For this review, take the finished solid that the model builds, in its own axes (mm). A direction names the side the tool comes from. Round coordinates to 2 decimals unless told otherwise and drop trailing zeros. Write each loop counter-clockwise with the first axis right and the second up, starting at its lowest first coordinate (ties: lowest second). Pieces come first, ordered by that corner, then holes. Notation, with made-up numbers: M -5.5,4 L 19.5,4 A30 ccw 19.5,40 Z; hole C 68,76.5 d7. An arc over 180 degrees is marked long. Use one line per item in the form item = value. Start each with the question number.
Item 1: Add section D-D (z = -2.2). State the section outline as (x, y) points, and give its area (3 significant figures).
Item 2: For faces 1 (the flat face through (1.25, 16, 0)), 2 (the flat face through (0, 0, 0)), 3 (the flat face through (1.2, 14, 1.2)), list the 3-axis set-ups (+Z, -Z, +X, -X, +Y, -Y) from which the entire face can be reached by the end or side of a thin tool; tool diameter is ignored.
Item 3: Add section A-A (z = 0). State the section outline as (x, y) points, and give its area (4 significant figures).
Item 4: For line 1 (Y direction, x = 0.55, z = 0.5); line 2 (Y direction, x = -0.8, z = -1.85); line 3 (X direction, y = 13, z = 0.4), list the stretches that pass through material, from the lowest coordinate up. Write a range as [from, to].
Item 5: Add section B-B (y = 4.75). State the section outline as (x, z) points, and give its area (3 significant figures).
Item 6: Add section C-C (x = -1.9). State the section outline as (y, z) points, and give its area (3 significant figures).
Item 7: Draft analysis for pull direction X (two halves, no side actions). For faces 4 (the flat face through (0.616, 16.014, -1.088)), 5 (the flat face through (-1.25, 16, 0)), 6 (the flat face through (0.6, 17, -1.3)), 7 (the cylindrical face through (1.5, 7.16, -0.07)), state which applies: released by +X, released by -X, zero draft, split by the parting line, or undercut.
Item 8: For P1, Ø1.5, axis at y = 8, z = 2, coming from the +X side; P2, Ø1, axis at y = 4, z = -0.5, coming from the -X side, all flat-tipped, find the tip position at first contact; note any pin that passes through.
Autodesk Inventor part; units mm, degrees
ref_plane "YZ Plane" through (0, 0, 0) normal (1, 0, 0) x (0, 1, 0)
ref_plane "XZ Plane" through (0, 0, 0) normal (0, 1, 0) x (-1, 0, 0)
ref_plane "XY Plane" through (0, 0, 0) normal (0, 0, 1) x (1, 0, 0)
sketch "Sketch1" plane through (0, 0, 0) normal (0, 1, 0) x (-1, 0, 0)
  circle A0 centre (0, 0) radius 1.5
  dimension "d0" = 3
extrude "Extrusion1" add sketch "Sketch1" along normal blind 14
sketch "Sketch2" plane through (0, 14, 0) normal (0, 1, 0) x (1, 0, 0)
  circle A0 centre (0, 0) radius 1.5
  circle A1 centre (0, 0) radius 2.75
  dimension "d3" = 5.5
extrude "Extrusion2" add sketch "Sketch2" along normal blind 3 contours A0 | A1
sketch "Sketch3" plane through (0, 17, 0) normal (0, 1, 0) x (1, 0, 0)
  circle A0 centre (0, 0) radius 2.75
  line L0 (0, 1.4434) -> (1.25, 0.7217)
  line L1 (1.25, 0.7217) -> (1.25, -0.7217)
  line L2 (1.25, -0.7217) -> (0, -1.4434)
  line L3 (0, -1.4434) -> (-1.25, -0.7217)
  line L4 (-1.25, -0.7217) -> (-1.25, 0.7217)
  line L5 (-1.25, 0.7217) -> (0, 1.4434)
  dimension "d6" = 2.5
extrude "Extrusion3" cut sketch "Sketch3" against normal blind 2 contours L0 L1 L2 L3 L4 L5
thread "Thread1"
chamfer "Chamfer1" distance 0.5 angle 45 1 edges at (1.5, 0, 0)
properties part number "M3x14SHCS"
Calculated:
q1.outline = M -1.65,14 L 1.65,14 L 1.65,17 L -1.65,17 Z
q1.area = 9.90 mm^2
q2.face_1 = +Y
q2.face_2 = +Z, -Z, +X, -X, -Y
q2.face_3 = -Y
q3.outline = M -2.75,14 L -1.5,14 L -1.5,0.5 L -1,0 L 1,0 L 1.5,0.5 L 1.5,14 L 2.75,14 L 2.75,17 L 1.25,17 L 1.25,15 L -1.25,15 L -1.25,17 L -2.75,17 Z
q3.area = 53.25 mm^2
q4.line_1 = [0, 15]
q4.line_2 = [14, 17]
q4.line_3 = [-1.45, 1.45]
q5.outline = C 0,0 d3
q5.area = 7.07 mm^2
q6.outline = M 14,-1.99 L 17,-1.99 L 17,1.99 L 14,1.99 Z
q6.area = 11.9 mm^2
q7.face_4 = undercut
q7.face_5 = undercut
q7.face_6 = zero draft
q7.face_7 = split by the parting line
q8.P1 = 0.83
q8.P2 = -1.5
